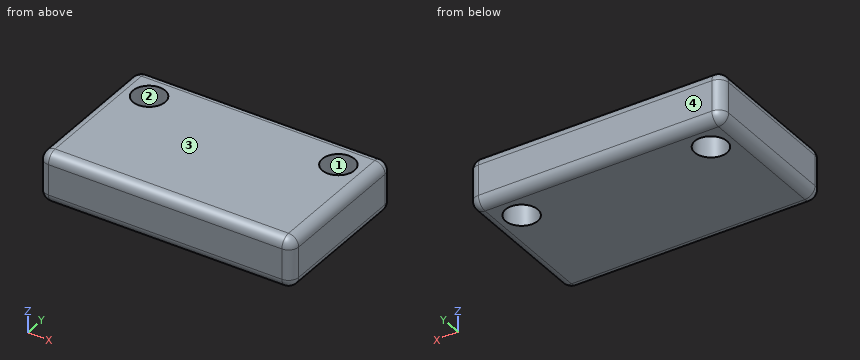
from build123d import *

# Parameters (mm, degrees)
ESBO_O1_W                = 25
ESBO_O1_H                = 15
RESSALTO_EXTRUS_O1_DEPTH = 5
ESBO_O2_R                = 1.5875
CORTE_EXTRUS_O1_DEPTH    = 16.411035007
FILETE2_R                = 1


with BuildPart() as part:
    # Esboço1 → Ressalto-extrusão1 (new body)
    with BuildSketch(Plane.XY):
        Rectangle(ESBO_O1_W, ESBO_O1_H)
    extrude(amount=RESSALTO_EXTRUS_O1_DEPTH)

    # Esboço2 → Corte-extrusão1 (cut, through all)
    with BuildSketch(Plane.XY.offset(5)):
        with Locations((-9.325, 4.325)):
            Circle(ESBO_O2_R)
        with Locations((9.325, 4.325)):
            Circle(ESBO_O2_R)
    extrude(amount=-CORTE_EXTRUS_O1_DEPTH, mode=Mode.SUBTRACT)

    # Filete2
    filete2_edges = [part.edges().sort_by_distance(p)[0] for p in [
        (12.5, 0, 5),
        (0, 7.5, 5),
        (-12.5, 0, 5),
        (0, 7.5, 0),
        (12.5, 0, 0),
        (0, -7.5, 0),
        (-12.5, 0, 0),
        (0, -7.5, 5),
        (-12.5, 7.5, 2.5),
        (12.5, 7.5, 2.5),
        (12.5, -7.5, 2.5),
        (-12.5, -7.5, 2.5),
    ]]
    fillet(filete2_edges, radius=FILETE2_R)


solid = part.part
Verification items for the finished model (mm, model axes). Face numbers are marked on the shaded views. Give positions to 0.01 mm unless a question says otherwise; leave off trailing zeros. Loops run counter-clockwise (first coordinate to the right, second up) from the corner with the lowest first, then second, coordinate; pieces in that order, holes last. Notation, with made-up numbers: (2, 30.5) - (17, 30.5) arc R11 cw to (17, 34.5) - close; hole circle Ø2 at (81.25, -1.75). An arc over 180 degrees is marked (long way). Write each question's results on one line, items separated by ' | '.
1) Depth check by flat-ended pin: P1, Ø3, axis at x = -9.325, y = 4.325, coming from the -Z side (3 decimals). Enter the tip coordinate at first touch or a pass-through.
Solution:
P1: through
2) Sectioned sample at A-A on z = 1.45. Record the boundary of the cut face in (x, y) (1 decimal).
Solution:
outline: (-12.5, -6.5) arc R1 ccw to (-11.5, -7.5) - (11.5, -7.5) arc R1 ccw to (12.5, -6.5) - (12.5, 6.5) arc R1 ccw to (11.5, 7.5) - (-11.5, 7.5) arc R1 ccw to (-12.5, 6.5) - close; hole circle Ø3.2 at (-9.3, 4.3); hole circle Ø3.2 at (9.3, 4.3)
3) Sectioned sample at D-D on x = -8.5. Record the boundary of the cut face in (y, z).
Solution:
outline: (-7.5, 1) arc R1 ccw to (-6.5, 0) - (2.97, 0) - (2.97, 5) - (-6.5, 5) arc R1 ccw to (-7.5, 4) - close; (5.68, 0) - (6.5, 0) arc R1 ccw to (7.5, 1) - (7.5, 4) arc R1 ccw to (6.5, 5) - (5.68, 5) - close
4) Material ranges on L1, parallel to X at y = 3.5, z = 3.85; L2, parallel to X at y = 5.75, z = 2.65; L3, parallel to Y at x = 7.25, z = 0.75, recorded low to high. Write a range as from..to.
Solution:
L1: -12.5..-10.68, -7.97..7.97, 10.68..12.5 | L2: -12.5..-10.02, -8.63..8.63, 10.02..12.5 | L3: -7.47..7.47
5) Sectioned sample at B-B on x = 10.5. Record the boundary of the cut face in (y, z).
Solution:
outline: (-7.5, 1) arc R1 ccw to (-6.5, 0) - (3.26, 0) - (3.26, 5) - (-6.5, 5) arc R1 ccw to (-7.5, 4) - close; (5.39, 0) - (6.5, 0) arc R1 ccw to (7.5, 1) - (7.5, 4) arc R1 ccw to (6.5, 5) - (5.39, 5) - close
6) Sectioned sample at C-C on y = 6.75. Record the boundary of the cut face in (x, z), plus the area to 3 significant figures.
Solution:
outline: (-12.47, 1) arc R0.97 ccw to (-11.5, 0.03) - (11.5, 0.03) arc R0.97 ccw to (12.47, 1) - (12.47, 4) arc R0.97 ccw to (11.5, 4.97) - (-11.5, 4.97) arc R0.97 ccw to (-12.47, 4) - close | area: 122 mm2
7) Mould release check, pull along Y, two halves, no side actions. Record for the marked faces 1, 2, 3 and 4: pulls with the +Y half, pulls with the -Y half, needs draft (parallel to the pull), parting line crosses it, or undercut.
Solution:
face 1: undercut | face 2: undercut | face 3: needs draft | face 4: pulls with the +Y half
